CAD build for the part. Positions are in the model's coordinates, mm. A direction names the side the tool comes from. Round coordinates to 2 decimals unless told otherwise and drop trailing zeros. Loops run counter-clockwise (first coordinate to the right, second up) from the corner with the lowest first, then second, coordinate; pieces in that order, holes last.
```python
from build123d import *

# Parameters (mm, degrees)
SKETCH1_R           = 8.75
BOSS_EXTRUDE1_DEPTH = 15
SKETCH2_R           = 7
CUT_EXTRUDE1_DEPTH  = 8
CUT_EXTRUDE2_DEPTH  = 5.5
CHAMFER1_SIZE       = 1
CHAMFER2_SIZE       = 1


with BuildPart() as part:
    # Sketch1 → Boss-Extrude1 (new body)
    with BuildSketch(Plane(origin=(0, 0, 0), x_dir=(1, 0, 0), z_dir=(0, 1, 0))):
        with Locations(Location((0, 0, 0), (0, 0, 270))):
            Circle(SKETCH1_R)
    extrude(amount=BOSS_EXTRUDE1_DEPTH)

    # Sketch2 → Cut-Extrude1 (cut)
    with BuildSketch(Plane.XZ):
        with Locations(Location((0, 0, 0), (0, 0, 270))):
            Circle(SKETCH2_R)
    extrude(amount=-CUT_EXTRUDE1_DEPTH, mode=Mode.SUBTRACT)

    # Sketch3 → Cut-Extrude2 (cut)
    with BuildSketch(Plane.XZ.offset(-8)):
        with BuildLine():
            Line((-2.75, 1.732050808), (2.75, 1.732050808))
            ThreePointArc((2.75, 1.732050808), (0, -3.25), (-2.75, 1.732050808))
        make_face()
    extrude(amount=-CUT_EXTRUDE2_DEPTH, mode=Mode.SUBTRACT)

    # Chamfer1
    chamfer1_edges = [part.edges().sort_by_distance(p)[0] for p in [
        (0, 15, -8.75),
    ]]
    chamfer(chamfer1_edges, length=CHAMFER1_SIZE)

    # Chamfer2
    chamfer2_edges = [part.edges().sort_by_distance(p)[0] for p in [
        (0, 8, -3.25),
        (0, 8, 1.732050808),
    ]]
    chamfer(chamfer2_edges, length=CHAMFER2_SIZE)


solid = part.part
```
Item 1: Cut at A-A, the plane z = 0. Give the cut face in (x, y).
Answers follow:
outline: (-8.75, 0) - (-7, 0) - (-7, 8) - (-4.25, 8) - (-3.25, 9) - (-3.25, 13.5) - (3.25, 13.5) - (3.25, 9) - (4.25, 8) - (7, 8) - (7, 0) - (8.75, 0) - (8.75, 14) - (7.75, 15) - (-7.75, 15) - (-8.75, 14) - close
Item 2: Flat gauge pins, fed straight in: P1, Ø4, axis at y = 10.5, z = 5.5, coming from the -X side; P2, Ø1.3, axis at x = -1, y = 12, coming from the -Z side; P3, Ø3, axis at x = 2, z = -2.5, coming from the -Y side. Where does each tip first touch, or does it go through?
Answers follow:
P1: stops at x = -8.02
P2: stops at z = -8.74
P3: stops at y = 8
Item 3: Cut at D-D, the plane y = 10. Give the cut face in (x, z).
Answers follow:
outline: circle Ø17.5 at (0, 0); hole (-2.75, 1.73) arc R3.25 ccw (long way) to (2.75, 1.73) - close
Item 4: 3-axis set-ups, long thin cutter, end or side, ignore diameter. For faces 1 (the flat face through (0, 15, 0)), 2 (the flat face through (-0.046, 8.507, 2.225)): which of +Z, -Z, +X, -X, +Y, -Y reach the whole face in a straight line?
Answers follow:
face 1: +Z, -Z, +X, -X, +Y
face 2: -Y
Item 5: Probe line 1 (X direction, y = 12, z = 0); line 2 (X direction, y = 6, z = 0); line 3 (Y direction, x = -4.5, z = 2.25). List the from-to ranges inside material, lowest first.
Answers follow:
line 1: x = -8.75 to -3.25, 3.25 to 8.75
line 2: x = -8.75 to -7, 7 to 8.75
line 3: y = 8 to 15
Item 6: Two-plate mould, pull along Z, no slides. Class faces 3 (the cylindrical face through (-6.834, 3.944, 1.517)), 4 (the flat face through (6, 0, -4)), 5 (the flat face through (0, 11, 1.732)), 6 (the cylindrical face through (-5.324, 6.902, -6.944)): released by +Z, released by -Z, zero draft, split by the parting line, or undercut.
Answers follow:
face 3: undercut
face 4: zero draft
face 5: undercut
face 6: split by the parting line
Item 7: Cut at C-C, the plane y = 6.5. Give the cut face in (x, z).
Answers follow:
outline: circle Ø17.5 at (0, 0); hole circle Ø14 at (0, 0)
Item 8: Cut at B-B, the plane x = 0. Give the cut face in (y, z), plus the area to 3 significant figures.
Answers follow:
outline: (0, -8.75) - (14, -8.75) - (15, -7.75) - (15, 7.75) - (14, 8.75) - (0, 8.75) - (0, 7) - (8, 7) - (8, 2.73) - (9, 1.73) - (13.5, 1.73) - (13.5, -3.25) - (9, -3.25) - (8, -4.25) - (8, -7) - (0, -7) - close
area: 121 mm2
